```python
from build123d import *

# Parameters (mm, degrees)
SKETCH_2_W      = 100.501056251
SKETCH_2_H      = 149.951645819
SKETCH_2_R      = 1.6
EXTRUDE_1_DEPTH = 3


with BuildPart() as part:
    # 草图2 → 凸台-拉伸1 (new body)
    with BuildSketch(Plane(origin=(58.724000156, 80.989637793, 0), x_dir=(0.8095795047809408, -0.5870102430440604, 0), z_dir=(0.5870102430440604, 0.8095795047809408, 0))):
        with Locations((-8.300782896, -27.864106314)):
            Rectangle(SKETCH_2_W, SKETCH_2_H)
        with Locations(Location((-45.551311022, 43.111716595, 0), (0, 0, 180))):
            Circle(SKETCH_2_R, mode=Mode.SUBTRACT)
        with Locations(Location((-37.551311022, 43.111716595, 0), (0, 0, 180))):
            Circle(SKETCH_2_R, mode=Mode.SUBTRACT)
        with Locations(Location((20.949745229, 43.111716595, 0), (0, 0, 180))):
            Circle(SKETCH_2_R, mode=Mode.SUBTRACT)
        with Locations(Location((28.949745229, 43.111716595, 0), (0, 0, 180))):
            Circle(SKETCH_2_R, mode=Mode.SUBTRACT)
        with Locations((28.949745229, -98.839929224)):
            Circle(SKETCH_2_R, mode=Mode.SUBTRACT)
        with Locations((20.949745229, -98.839929224)):
            Circle(SKETCH_2_R, mode=Mode.SUBTRACT)
        with Locations((-37.551311022, -98.839929224)):
            Circle(SKETCH_2_R, mode=Mode.SUBTRACT)
        with Locations((-45.551311022, -98.839929224)):
            Circle(SKETCH_2_R, mode=Mode.SUBTRACT)
    extrude(amount=-EXTRUDE_1_DEPTH)


solid = part.part
```
Here's how the part is built. I have some questions about the finished solid (model axes, mm). Coordinates: 2 decimals unless noted, no trailing zeros. Loops run counter-clockwise (first coordinate to the right, second up) from the corner with the lowest first, then second, coordinate; pieces in that order, holes last. Notation, with made-up numbers: (22, 50) - (63, 50) arc R18 cw to (63, 78) - close; hole circle Ø3 at (26, -40). An arc over 180 degrees is marked (long way). Answer as CSV lines item,"result".
Q1. If we section it at A-A, the plane z = -26: Write out the boundary of the cut face in (x, y).
Response:
outline,"(9.56, 112.93) - (90.92, 53.94) - (92.69, 56.36) - (11.32, 115.36) - close"
Q2. If we section it at B-B, the plane x = 68.5: Write out the boundary of the cut face in (y, z).
Response:
outline,"(70.2, -47.11) - (73.9, -47.11) - (73.9, 102.84) - (70.2, 102.84) - close"
Q3. We'd pull the mould along Y, two halves only. Please class faces 1 (the face through (49.67, 83.85, 26.81)), 2 (the face through (20.381, 106.965, -44.531)), 3 (the face through (51, 85, 102.84)): pulls with the +Y half, pulls with the -Y half, needs draft (parallel to the pull), parting line crosses it, or undercut.
Response:
face 1,"pulls with the -Y half"
face 2,"undercut"
face 3,"needs draft"
Q4. If I drill on L1, parallel to X at y = 78, z = 26; L2, parallel to Y at x = 22, z = 95.5; L3, parallel to X at y = 91, z = -21.5, over which ranges is the centre line in solid material (lowest first)? Write a range as [from, to].
Response:
L1,"[57.74, 62.85]"
L2,"[103.91, 107.62]"
L3,"[39.81, 44.92]"
Q5. For pin 1 (3 mm diameter, centred on x = 18.5, z = 54, fed in from -Y); pin 2 (2 mm diameter, centred on y = 106, z = 57, fed in from -X); pin 3 (6 mm diameter, centred on y = 84.5, z = 66, fed in from -X), each with a flat end and sliding along its axis, tell me the tip position at first contact or that it passes through.
Response:
pin 1,"y = 105.36"
pin 2,"x = 17.74"
pin 3,"x = 44.63"
